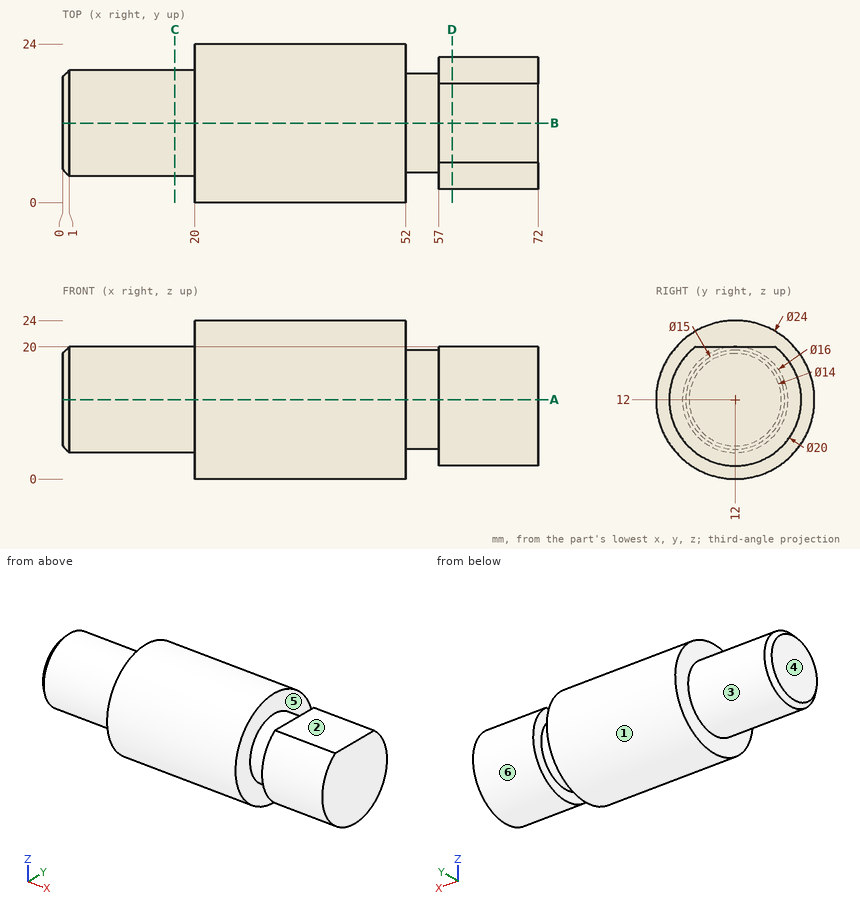
The figure shows three views and two pictorial views of one solid part (mm, origin at its lowest corner). Answer the questions. A direction names the side the tool comes from. Round coordinates to 2 decimals unless told otherwise and drop trailing zeros. Write each loop counter-clockwise with the first axis right and the second up, starting at its lowest first coordinate (ties: lowest second). Pieces come first, ordered by that corner, then holes. Notation, with made-up numbers: (53.5, 13) -> (64.5, 13) arc R12 ccw to (64.5, 31) -> close; hole circle Ø11 at (48, 27). An arc over 180 degrees is marked (long way). Answer as a JSON object with one key per item and string values. Group by question number.
Q1. Each of these flat-tipped pins is pushed along its axis until it touches: pin 1 Ø5 at (x, z) = (38.5, 14.5) entering from -Y; pin 2 Ø4 at (x, z) = (41, 7.5) entering from +Y; pin 3 Ø10 at (x, z) = (62.5, 19) entering from -Y; pin 4 Ø6 at (x, y) = (58.5, 11) entering from +Z. Where does it stop, or does it pass through?
Q2. Determine the mould class of the marked faces 4, 5 and 6 for opening direction X: pulls with the +X half, pulls with the -X half, needs draft (parallel to the pull), parting line crosses it, or undercut.
Q3. Straight lines are drawn through the part: line 1 along X through (y, z) = (17.5, 4.5); line 2 along X through (y, z) = (13, 22.5); line 3 along X through (y, z) = (19.75, 13.75). For each, find the intervals that lie inside material, in ascending order.
Q4. Section B-B (y = 12) is taken. Write down the section's boundary in (x, z).
Q5. Section C-C (x = 17) is taken. Write down the section's boundary in (y, z).
Q6. Section D-D (x = 59) is taken. Write down the section's boundary in (y, z), plus the area to 3 significant figures.
Q7. Which of the six approach directions +Z, -Z, +X, -X, +Y, -Y give full straight-line access (tool end or side, diameter ignored) to the marked faces 1, 2 and 3?
Q8. Section A-A (z = 12) is taken. Write down the section's boundary in (x, y).
Check values:
{
 "1": {"pin 1": "y = 0", "pin 2": "y = 23.74", "pin 3": "y = 2.2", "pin 4": "z = 20"},
 "2": {"face 4": "pulls with the -X half", "face 5": "undercut", "face 6": "needs draft"},
 "3": {"line 1": "20 to 52, 57 to 72", "line 2": "20 to 52", "line 3": "0.95 to 52, 57 to 72"},
 "4": {"outline": "(0, 5) -> (1, 4) -> (20, 4) -> (20, 0) -> (52, 0) -> (52, 4.5) -> (57, 4.5) -> (57, 2) -> (72, 2) -> (72, 20) -> (57, 20) -> (57, 19.5) -> (52, 19.5) -> (52, 24) -> (20, 24) -> (20, 20) -> (1, 20) -> (0, 19) -> close"},
 "5": {"outline": "circle Ø16 at (12, 12)"},
 "6": {"outline": "(6, 20) arc R10 ccw (long way) to (18, 20) -> close", "area": "298 mm^2"},
 "7": {"face 1": "+X, -X", "face 2": "+Z, +X, +Y, -Y", "face 3": "-X"},
 "8": {"outline": "(0, 5) -> (1, 4) -> (20, 4) -> (20, 0) -> (52, 0) -> (52, 4.5) -> (57, 4.5) -> (57, 2) -> (72, 2) -> (72, 22) -> (57, 22) -> (57, 19.5) -> (52, 19.5) -> (52, 24) -> (20, 24) -> (20, 20) -> (1, 20) -> (0, 19) -> close"}
}
